```python
from build123d import *

# Parameters (mm, degrees)
SKETCH1_R           = 38.1
BOSS_EXTRUDE1_DEPTH = 4.826
SKETCH2_R           = 38.1
BOSS_EXTRUDE2_DEPTH = 3.302
BOSS_EXTRUDE2_DRAFT = -70
SKETCH3_R           = 47.172170439
BOSS_EXTRUDE3_DEPTH = 3.81
SKETCH4_R           = 46.472170439
CUT_EXTRUDE1_DEPTH  = 0.2
SKETCH6_R           = 34.772170439
SKETCH6_R_2         = 11.35
CUT_EXTRUDE2_DEPTH  = 2.7
SKETCH7_R           = 5.35
CUT_EXTRUDE3_DEPTH  = 68.736312063
SKETCH8_R           = 11.35
SKETCH8_R_2         = 5.35
BOSS_EXTRUDE4_DEPTH = 50.8
SKETCH9_R           = 7.35
CUT_EXTRUDE4_DEPTH  = 3
CUT_EXTRUDE5_START  = -3
SKETCH10_R          = 7.35
CUT_EXTRUDE5_DEPTH  = 3
SKETCH12_R          = 6.4
CUT_EXTRUDE8_DEPTH  = 83.032578722
SKETCH13_R          = 6.4
CUT_EXTRUDE9_DEPTH  = 80.227293099


with BuildPart() as part:
    # Sketch1 → Boss-Extrude1 (new body)
    with BuildSketch(Plane(origin=(0, 0, 0), x_dir=(1, 0, 0), z_dir=(0, 1, 0))):
        with Locations(Location((0, 0, 0), (0, 0, 270))):
            Circle(SKETCH1_R)
    extrude(amount=BOSS_EXTRUDE1_DEPTH)


with BuildPart() as boss_extrude2_tool:
    # Sketch2 → Boss-Extrude2 (with draft: the straight prism first)
    with BuildSketch(Plane(origin=(0, 4.826, 0), x_dir=(1, 0, 0), z_dir=(0, 1, 0))):
        with Locations(Location((0, 0, 0), (0, 0, 270))):
            Circle(SKETCH2_R)
    extrude(amount=BOSS_EXTRUDE2_DEPTH)
    # Boss-Extrude2: the draft: its side faces are tilted about the plane it starts from
    boss_extrude2_sides = [boss_extrude2_tool.faces().sort_by_distance(p)[0] for p in [
        (0, 6.477, -38.1),
    ]]
    draft(boss_extrude2_sides, Plane(origin=(0, 4.826, 0), x_dir=(1, 0, 0), z_dir=(0, 1, 0)), BOSS_EXTRUDE2_DRAFT)


with BuildPart() as part_1:
    add(part.part)

    # Boss-Extrude2: add boss_extrude2_tool
    add(boss_extrude2_tool.part)

    # Sketch3 → Boss-Extrude3 (add)
    with BuildSketch(Plane(origin=(0, 8.128, 0), x_dir=(1, 0, 0), z_dir=(0, 1, 0))):
        with Locations(Location((0, 0, 0), (0, 0, 90))):
            Circle(SKETCH3_R)
    extrude(amount=BOSS_EXTRUDE3_DEPTH)

    # Sketch4 → Cut-Extrude1 (cut)
    with BuildSketch(Plane(origin=(0, 11.938, 0), x_dir=(1, 0, 0), z_dir=(0, 1, 0))):
        with Locations(Location((0, 0, 0), (0, 0, 270))):
            Circle(SKETCH4_R)
    extrude(amount=-CUT_EXTRUDE1_DEPTH, mode=Mode.SUBTRACT)

    # Sketch6 → Cut-Extrude2 (cut)
    with BuildSketch(Plane(origin=(0, 11.738, 0), x_dir=(1, 0, 0), z_dir=(0, 1, 0))):
        with Locations(Location((0, 0, 0), (0, 0, 270))):
            Circle(SKETCH6_R)
        with Locations(Location((0, 0, 0), (0, 0, 270))):
            Circle(SKETCH6_R_2, mode=Mode.SUBTRACT)
    extrude(amount=-CUT_EXTRUDE2_DEPTH, mode=Mode.SUBTRACT)

    # Sketch7 → Cut-Extrude3 (cut, through all)
    with BuildSketch(Plane(origin=(0, 11.738, 0), x_dir=(1, 0, 0), z_dir=(0, 1, 0))):
        with Locations(Location((0, 0, 0), (0, 0, 270))):
            Circle(SKETCH7_R)
    extrude(amount=-CUT_EXTRUDE3_DEPTH, mode=Mode.SUBTRACT)

    # Sketch8 → Boss-Extrude4 (add)
    with BuildSketch(Plane.XZ):
        with Locations(Location((0, 0, 0), (0, 0, 90))):
            Circle(SKETCH8_R)
        with Locations(Location((0, 0, 0), (0, 0, 90))):
            Circle(SKETCH8_R_2, mode=Mode.SUBTRACT)
    extrude(amount=BOSS_EXTRUDE4_DEPTH)

    # Sketch9 → Cut-Extrude4 (cut)
    with BuildSketch(Plane.XZ.offset(50.8)):
        with Locations(Location((0, 0, 0), (0, 0, 270))):
            Circle(SKETCH9_R)
    extrude(amount=-CUT_EXTRUDE4_DEPTH, mode=Mode.SUBTRACT)

    # Sketch10 → Cut-Extrude5 (cut)
    with BuildSketch(Plane(origin=(0, 11.738, 0), x_dir=(1, 0, 0), z_dir=(0, 1, 0)).offset(CUT_EXTRUDE5_START)):
        with Locations(Location((0, 0, 0), (0, 0, 90))):
            Circle(SKETCH10_R)
    extrude(amount=CUT_EXTRUDE5_DEPTH, mode=Mode.SUBTRACT)

    # Sketch12 → Cut-Extrude8 (cut, through all)
    with BuildSketch(Plane(origin=(0, -35.8, 0), x_dir=(-1, 0, 0), z_dir=(0, -1, 0))):
        with Locations(Location((0, 0, 0), (0, 0, 90))):
            Circle(SKETCH12_R)
    extrude(amount=CUT_EXTRUDE8_DEPTH, mode=Mode.SUBTRACT)

    # Sketch13 → Cut-Extrude9 (cut, through all)
    with BuildSketch(Plane(origin=(0, -30.8, 0), x_dir=(-1, 0, 0), z_dir=(0, -1, 0))):
        with Locations(Location((0, 0, 0), (0, 0, 90))):
            Circle(SKETCH13_R)
    extrude(amount=-CUT_EXTRUDE9_DEPTH, mode=Mode.SUBTRACT)


solid = part_1.part
```
CAD build for the part. Positions are in the model's coordinates, mm. A direction names the side the tool comes from. Round coordinates to 2 decimals unless told otherwise and drop trailing zeros. Loops run counter-clockwise (first coordinate to the right, second up) from the corner with the lowest first, then second, coordinate; pieces in that order, holes last. Notation, with made-up numbers: M -22.75,36.5 L 11.25,36.5 A17 ccw 11.25,49.5 Z; hole C 65.25,-29.5 d8. An arc over 180 degrees is marked long. Return JSON: item names as keys, results as strings. Group by question number.
(1) Wall check: probe 1 along X at (y, z) = (-32, 0); probe 2 along X at (y, z) = (-49, 0); probe 3 along Y at (x, z) = (-8, 6). Give the ranges that are in metal, low to high. Write a range as [from, to].
(2) Mould opens along Z. For faces 1 (the cylindrical face through (6.906, -25.044, -9.007)), 2 (the cylindrical face through (-7.175, -49.321, 1.593)), 3 (the flat face through (9, 0, 8)), 4 (the flat face through (7, -47.8, -1)) say: +Z half, -Z half, draft (parallel to the pull), parting line (faces both ways), or undercut.
(3) Saw through at A-A, the plane y = -9.5. List the corners of the cut face in (x, z), and give its area (3 significant figures).
(4) Tool access for faces 5 (the cylindrical face through (-3.89, -11.31, 5.08)), 6 (the cylindrical face through (-3.89, -41.72, 5.08)), 7 (the cylindrical face through (-2.074, 10.006, 47.127)): list every direction of +Z, -Z, +X, -X, +Y, -Y with a clear straight run to the whole face (end or side of a thin tool).
(5) Drop flat-ended pins along their axis: P1, Ø10, axis at x = 11, z = 24, coming from the +Y side; P2, Ø12, axis at y = -22, z = 17.5, coming from the +X side (3 decimals); P3, Ø10, axis at x = 27, z = -17, coming from the -Y side; P4, Ø12, axis at y = -15, z = -14, coming from the +X side. Give the stop position or say it passes through.
Answer list:
{
 "1": {"probe 1": "[-11.35, -5.35], [5.35, 11.35]", "probe 2": "[-11.35, -7.35], [7.35, 11.35]", "probe 3": "[-50.8, 11.74]"},
 "2": {"face 1": "parting line", "face 2": "undercut", "face 3": "draft", "face 4": "undercut"},
 "3": {"outline": "C 0,0 d22.7; hole C 0,0 d12.8", "area": "276 mm2"},
 "4": {"face 5": "+Y", "face 6": "-Y", "face 7": "+Y, -Y"},
 "5": {"P1": "y = 9.04", "P2": "through", "P3": "y = 0", "P4": "x = 8.05"}
}
